For this review, use the dimensioned drawing (mm, ordinates from the lowest corner) and the shaded views. A direction names the side the tool comes from. Give positions to 0.01 mm unless a question says otherwise; leave off trailing zeros. Write each loop counter-clockwise with the first axis right and the second up, starting at its lowest first coordinate (ties: lowest second). Pieces come first, ordered by that corner, then holes. Notation, with made-up numbers: (73, 18.5) -> (132, 18.5) arc R27 cw to (132, 57.5) -> close; hole circle Ø11 at (44.25, 38.5). An arc over 180 degrees is marked (long way). Return JSON: item names as keys, results as strings.
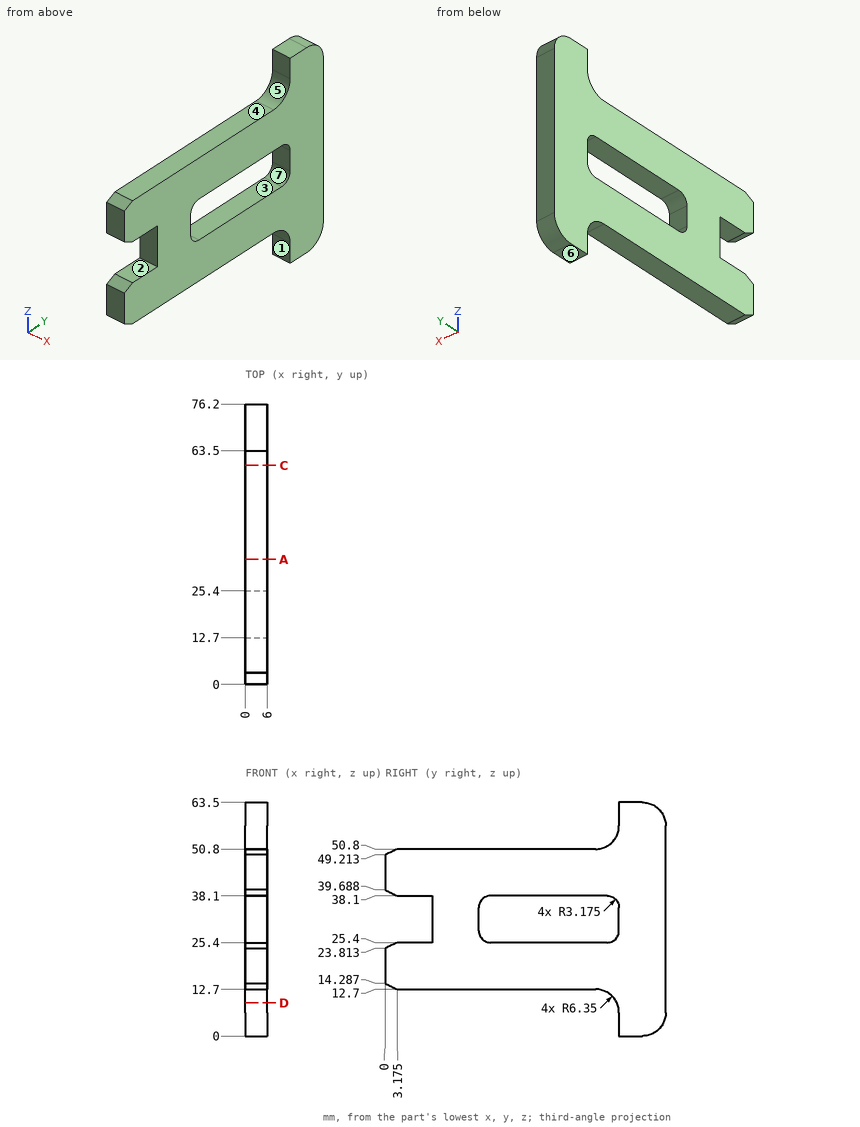
1. Add section D-D, the plane z = 9. State the section outline as (x, y) points.
Results found:
{"outline": "(0, 62.92) -> (6, 62.92) -> (6, 76.2) -> (0, 76.2) -> close"}
2. Add section A-A, the plane y = 34. State the section outline as (x, z) points, plus the area to 3 significant figures.
Results found:
{"outline": "(0, 12.7) -> (6, 12.7) -> (6, 25.4) -> (0, 25.4) -> close; (0, 38.1) -> (6, 38.1) -> (6, 50.8) -> (0, 50.8) -> close", "area": "152 mm²"}
3. For pin 1 (1 mm diameter, centred on x = 4, y = 22, fed in from -Z); pin 2 (2 mm diameter, centred on x = 1.5, y = 54, fed in from +Z); pin 3 (1.8 mm diameter, centred on x = 3, z = 60, fed in from -Y), all flat-tipped, find the tip position at first contact; note any pin that passes through.
Results found:
{"pin 1": "stops at z = 12.7", "pin 2": "stops at z = 50.8", "pin 3": "stops at y = 63.5"}
4. Add section C-C, the plane y = 59.5. State the section outline as (x, z) points.
Results found:
{"outline": "(0, 12.25) -> (6, 12.25) -> (6, 25.4) -> (0, 25.4) -> close; (0, 38.1) -> (6, 38.1) -> (6, 51.25) -> (0, 51.25) -> close"}
5. The part is to be moulded in two halves that separate along Y. For the marked faces 5, 6 and 7, say which applies: +Y half, -Y half, draft (parallel to the pull), parting line (faces both ways), or undercut.
Results found:
{"face 5": "-Y half", "face 6": "draft", "face 7": "undercut"}
6. For the marked faces 1, 2, 3 and 4, list the 3-axis set-ups (+Z, -Z, +X, -X, +Y, -Y) from which the entire face can be reached by the end or side of a thin tool; tool diameter is ignored.
Results found:
{"face 1": "-Z, +X, -X, -Y", "face 2": "+X, -X, -Y", "face 3": "+X, -X", "face 4": "+Z, +X, -X, -Y"}
7. To check wall thickness, follow probe 1 along Z at (x, y) = (3.1, 5); probe 2 along Y at (x, z) = (4.85, 28.5); probe 3 along Z at (x, y) = (5, 20). State the ranges of each line that lie inside material, in increasing order.
Results found:
{"probe 1": "z = 12.7 to 25.4, 38.1 to 50.8", "probe 2": "y = 12.7 to 25.4, 63.5 to 76.2", "probe 3": "z = 12.7 to 50.8"}
